Design review of the part shown in the three views and the two pictorial views. Dimensions are in mm from the part's minimum x, y and z. Give positions to 0.01 mm unless a question says otherwise; leave off trailing zeros. Order: outer loops, then holes, each group sorted by start corner. A loop starts at its lowest first (then second) coordinate and runs counter-clockwise, first axis right, second up. Notation, with made-up numbers: (64, -0.75) - (121, -0.75) arc R17 ccw to (121, 29.25) - close; hole circle Ø6 at (38, 22). An arc over 180 degrees is marked (long way). Put each result on its own line as item: value. Start each with the question number.
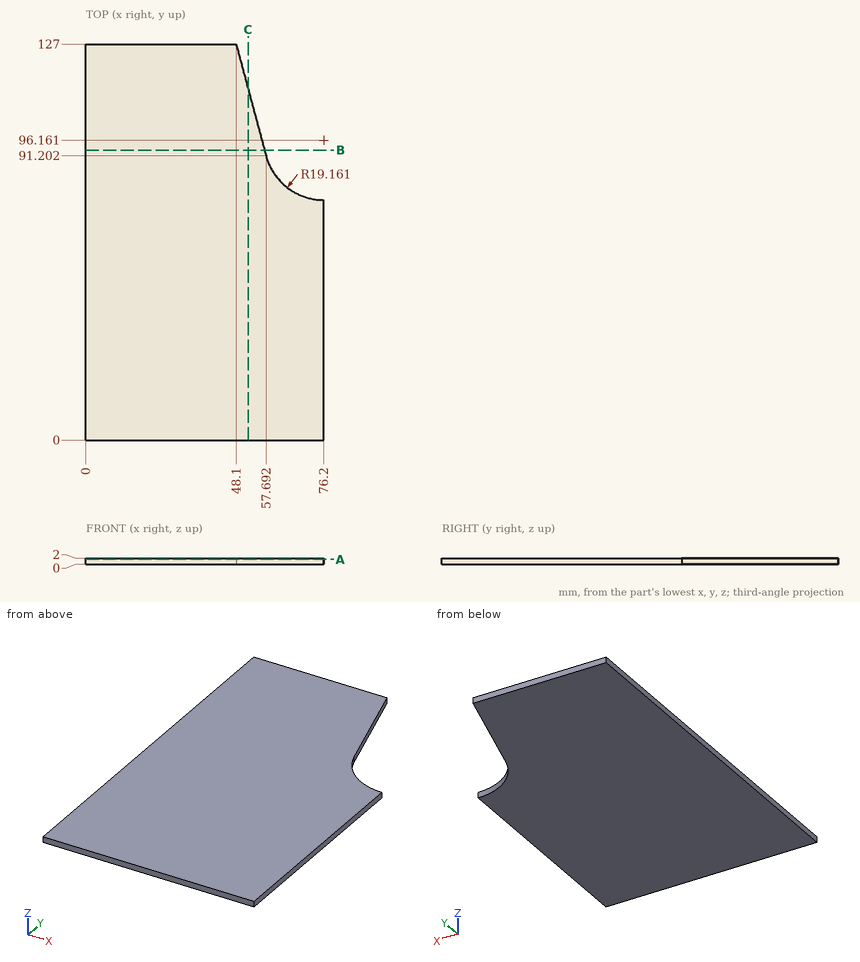
1. Add section A-A, the plane z = 1.6. Give the boundary of the cut face in (x, y), then the cut area to 3 significant figures.
2. Add section C-C, the plane x = 52. Give the boundary of the cut face in (y, z) (1 decimal).
3. Add section B-B, the plane y = 93. Give the boundary of the cut face in (x, z).
4. Wall thickness on line 1 (X direction, y = 118, z = 1.5); line 2 (X direction, y = 98, z = 1.4); line 3 (Y direction, x = 60.5, z = 0.25) (1 decimal): over which ranges is each line inside the solid? List them lowest first. Write a range as from..to.
5. Clearance check with a flat-ended pin moving along its axis: pin 1 (10 mm diameter, centred on x = 8, y = 97.5, fed in from -Z). State where the tip first meets the part, or that it passes through.
Found:
1. outline: (0, 0) - (76.2, 0) - (76.2, 77) arc R19.16 cw to (57.69, 91.2) - (48.1, 127) - (0, 127) - close
1. area: 8,650 mm^2
2. outline: (0, 0) - (112.4, 0) - (112.4, 2) - (0, 2) - close
3. outline: (0, 0) - (57.21, 0) - (57.21, 2) - (0, 2) - close
4. line 1: x = 0..50.51
4. line 2: x = 0..55.87
4. line 3: y = 0..85.2
5. pin 1: stops at z = 0
